Design review of the part shown in the three views and the two pictorial views. Dimensions are in mm from the part's minimum x, y and z. A direction names the side the tool comes from. Round coordinates to 2 decimals unless told otherwise and drop trailing zeros. Order: outer loops, then holes, each group sorted by start corner. A loop starts at its lowest first (then second) coordinate and runs counter-clockwise, first axis right, second up.
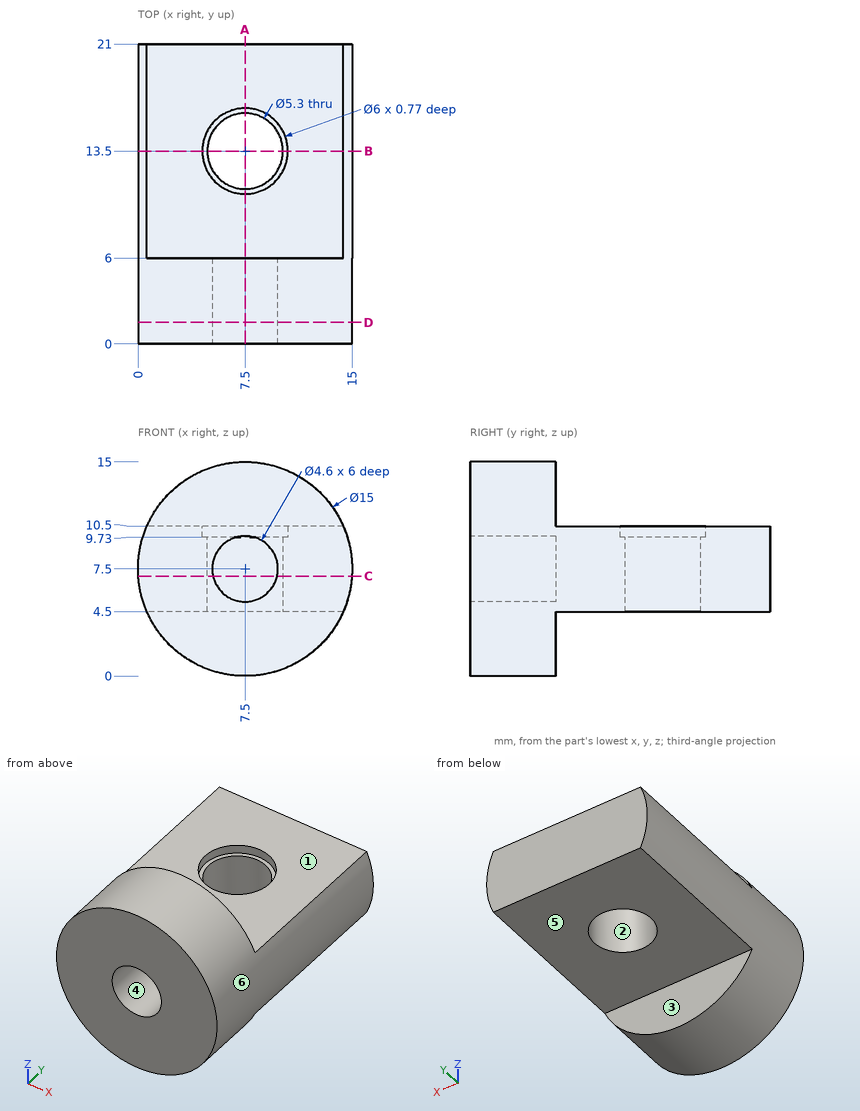
(1) Tool access review of the marked faces 1, 2 and 3: name each direction out of +Z, -Z, +X, -X, +Y, -Y from which nothing blocks a thin tool from reaching the whole face with its end or side.
(2) Wall thickness on L1, parallel to Z at x = 7.5, y = 3.7; L2, parallel to Y at x = 7.5, z = 8.35; L3, parallel to Y at x = 7.5, z = 10.25: over which ranges is each line inside the solid? List them lowest first.
(3) Draft analysis for pull direction X (two halves, no side actions). For the marked faces 4, 5 and 6, state which applies: pulls with the +X half, pulls with the -X half, needs draft (parallel to the pull), parting line crosses it, or undercut.
(4) Add section C-C on z = 7. Give the boundary of the cut face in (x, y) (3 decimals).
(5) Add section D-D on y = 1.5. Give the boundary of the cut face in (x, z).
(6) Add section A-A on x = 7.5. Give the boundary of the cut face in (y, z).
(7) Clearance check with flat-ended pins moving along their axes: P1, Ø1.8, axis at x = 6, y = 12.5, coming from the +Z side; P2, Ø5, axis at x = 5, y = 13, coming from the -Z side; P3, Ø3, axis at x = 8.5, y = 13, coming from the -Z side; P4, Ø1.5, axis at x = 6, y = 6.5, coming from the +Z side. State where each tip first meets the part, or that it passes through.
(8) Add section B-B on y = 13.5. Give the boundary of the cut face in (x, z).
Here are the results:
1. face 1: +Z, +X, -X, +Y
1. face 2: +Z, -Z
1. face 3: -Z, +X, -X, +Y
2. L1: z = 0 to 5.2, 9.8 to 15
2. L2: y = 6 to 10.85, 16.15 to 21
2. L3: y = 0 to 10.5, 16.5 to 21
3. face 4: undercut
3. face 5: needs draft
3. face 6: parting line crosses it
4. outline: (0.017, 0) - (5.255, 0) - (5.255, 6) - (9.745, 6) - (9.745, 0) - (14.983, 0) - (14.983, 21) - (0.017, 21) - close; hole circle Ø5.3 at (7.5, 13.5)
5. outline: circle Ø15 at (7.5, 7.5); hole circle Ø4.6 at (7.5, 7.5)
6. outline: (0, 0) - (6, 0) - (6, 4.5) - (10.85, 4.5) - (10.85, 9.73) - (10.5, 9.73) - (10.5, 10.5) - (6, 10.5) - (6, 15) - (0, 15) - (0, 9.8) - (6, 9.8) - (6, 5.2) - (0, 5.2) - close; (16.15, 4.5) - (21, 4.5) - (21, 10.5) - (16.5, 10.5) - (16.5, 9.73) - (16.15, 9.73) - close
7. P1: stops at z = 9.73
7. P2: stops at z = 4.5
7. P3: passes through
7. P4: stops at z = 14.94
8. outline: (0.63, 4.5) - (4.85, 4.5) - (4.85, 9.73) - (4.5, 9.73) - (4.5, 10.5) - (0.63, 10.5) arc R7.5 ccw to start; (10.15, 4.5) - (14.37, 4.5) arc R7.5 ccw to (14.37, 10.5) - (10.5, 10.5) - (10.5, 9.73) - (10.15, 9.73) - close
